Can you work these out from the drawing? Everything is in mm from the part's minimum corner. A direction names the side the tool comes from. Round coordinates to 2 decimals unless told otherwise and drop trailing zeros. Loops run counter-clockwise (first coordinate to the right, second up) from the corner with the lowest first, then second, coordinate; pieces in that order, holes last. Notation, with made-up numbers: (-9, -8) -> (48, -8) arc R18 ccw to (48, 17) -> close; hole circle Ø3 at (-8.5, 50.5). An arc over 180 degrees is marked (long way). One line per item, written item: value.
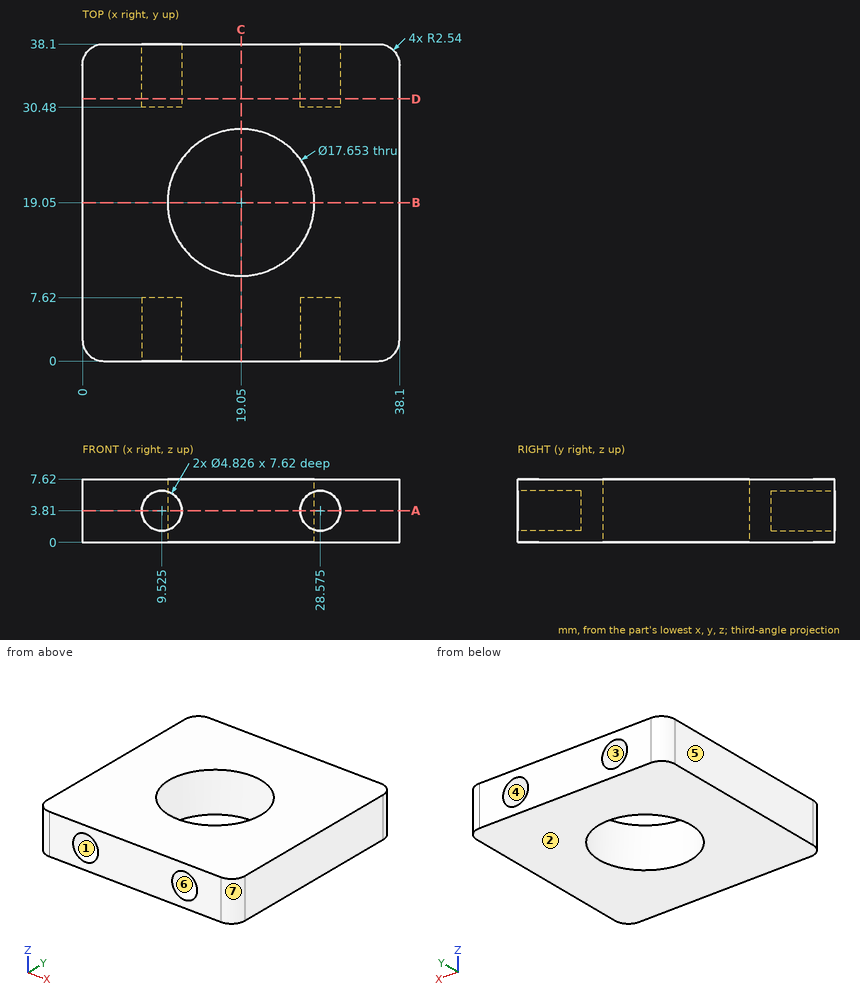
Item 1: If we section it at A-A on z = 3.81: List the corners of the cut face in (x, y) for me, plus the area to 3 significant figures.
Output:
outline: (0, 2.54) arc R2.54 ccw to (2.54, 0) -> (7.11, 0) -> (7.11, 7.62) -> (11.94, 7.62) -> (11.94, 0) -> (26.16, 0) -> (26.16, 7.62) -> (30.99, 7.62) -> (30.99, 0) -> (35.56, 0) arc R2.54 ccw to (38.1, 2.54) -> (38.1, 35.56) arc R2.54 ccw to (35.56, 38.1) -> (30.99, 38.1) -> (30.99, 30.48) -> (26.16, 30.48) -> (26.16, 38.1) -> (11.94, 38.1) -> (11.94, 30.48) -> (7.11, 30.48) -> (7.11, 38.1) -> (2.54, 38.1) arc R2.54 ccw to (0, 35.56) -> close; hole circle Ø17.65 at (19.05, 19.05)
area: 1,050 mm²
Item 2: For the marked faces 1, 2 and 3, which set-ups out of +Z, -Z, +X, -X, +Y, -Y let a thin tool reach every point of the face, with its end or its side?
Output:
face 1: -Y
face 2: -Z, +X, -X, +Y, -Y
face 3: +Y
Item 3: I need wall thicknesses on line 1 (X direction, y = 35.25, z = 3.81); line 2 (X direction, y = 4, z = 2); line 3 (X direction, y = 14.5, z = 2.25). Which ranges of each line are inside material? Lowest first, please. Write a range as from..to.
Output:
line 1: x = 0..7.11, 11.94..26.16, 30.99..38.1
line 2: x = 0..7.93, 11.12..26.98, 30.17..38.1
line 3: x = 0..11.49, 26.61..38.1
Item 4: Will these pins go through, and if not, where does the flat tip stop? pin 1 Ø3 at (x, z) = (12.5, 5) entering from -Y; pin 2 Ø3 at (x, z) = (9.525, 3.81) entering from -Y; pin 3 Ø4.5 at (x, z) = (28.575, 3.81) entering from +Y; pin 4 Ø14 at (x, y) = (19.05, 19.05) entering from -Z.
Output:
pin 1: stops at y = 0
pin 2: stops at y = 7.62
pin 3: stops at y = 30.48
pin 4: passes through
Item 5: If we section it at B-B on y = 19.05: List the corners of the cut face in (x, z) for me.
Output:
outline: (0, 0) -> (10.22, 0) -> (10.22, 7.62) -> (0, 7.62) -> close; (27.88, 0) -> (38.1, 0) -> (38.1, 7.62) -> (27.88, 7.62) -> close
Item 6: If we section it at D-D on y = 31.5: List the corners of the cut face in (x, z) for me (3 decimals), plus the area to 3 significant figures.
Output:
outline: (0, 0) -> (38.1, 0) -> (38.1, 7.62) -> (0, 7.62) -> close; hole circle Ø4.826 at (9.525, 3.81); hole circle Ø4.826 at (28.575, 3.81)
area: 254 mm²
Item 7: If we mould it in two halves opening along X, with no side actions, what happens to the marked faces 4, 5, 6 and 7? For each: released by +X, released by -X, zero draft, split by the parting line, or undercut.
Output:
face 4: undercut
face 5: released by -X
face 6: undercut
face 7: released by +X
